```python
from build123d import *

# Parameters (mm, degrees)
CUT_EXTRUDE2_REACH = 19.55
CIRPATTERN1_COUNT  = 12


with BuildPart() as part:
    # Sketch1 → Revolve1 (revolve)
    with BuildSketch(Plane.XY, mode=Mode.PRIVATE) as revolve1_sk:
        Polygon((3.937, 47.625), (3.937, 55.894079216), (0.8255, 55.894079216), (0.8255, 51.371485268), (2.7305, 51.371485268), (2.7305, 47.625), align=None)
    revolve(revolve1_sk.sketch.rotate(Axis((6.7945, 45.4025, 0), (0, 1, 0)), 270), axis=Axis((6.7945, 45.4025, 0), (0, 1, 0)))

    # Sketch2 → Cut-Extrude2 (cut, up to next)
    with BuildSketch(Plane(origin=(-1.519613368, 55.894079216, 0), x_dir=(-1, 0, 0), z_dir=(0, 1, 0)), mode=Mode.PRIVATE) as cut_extrude2_sk1:
        with BuildLine():
            Line((-3.694980373, 0.479092135), (-2.424980373, 0.973177048))
            ThreePointArc((-2.424980373, 0.973177048), (-2.345113368, 0), (-2.424980373, -0.973177048))
            Line((-2.424980373, -0.973177048), (-3.694980373, -0.479092135))
            Line((-3.694980373, -0.479092135), (-3.694980373, 0.479092135))
        make_face()
    cut_extrude2_tool1 = extrude(cut_extrude2_sk1.sketch, amount=-CUT_EXTRUDE2_REACH, mode=Mode.PRIVATE) & part.part
    cut_extrude2 = cut_extrude2_tool1.solids().sort_by_distance((1.436663, 55.894079, 0))[0]
    add(cut_extrude2, mode=Mode.SUBTRACT)

    # CirPattern1: Cut-Extrude2 ×12 about axis
    cirpattern1_axis = Axis((6.7945, 0, 0), (0, 1, 0))
    for i in range(1, CIRPATTERN1_COUNT):
        add(cut_extrude2.rotate(cirpattern1_axis, i * 360 / CIRPATTERN1_COUNT), mode=Mode.SUBTRACT)


solid = part.part
```
The model under review builds one solid part; all positions refer to its coordinate system, in mm. A direction names the side the tool comes from. Round coordinates to 2 decimals unless told otherwise and drop trailing zeros. Loops run counter-clockwise (first coordinate to the right, second up) from the corner with the lowest first, then second, coordinate; pieces in that order, holes last. Notation, with made-up numbers: M 53,35 L 82,35 A22 cw 82,42 Z; hole C 42,-16.75 d9. An arc over 180 degrees is marked long. Write item = value, one per line.
Item 1: Take a section at C-C on z = 3.5. Write out the cut boundary in (x, y) (3 decimals).
Return value:
outline = M 2.412,51.371 L 4.729,51.371 L 4.729,47.625 L 8.86,47.625 L 8.86,51.371 L 11.177,51.371 L 11.177,55.894 L 2.412,55.894 Z
Item 2: Take a section at D-D on y = 49.75. Write out the cut boundary in (x, z) (1 decimal).
Return value:
outline = C 6.8,0 d8.1; hole C 6.8,0 d5.7
Item 3: Insertion check: P1, Ø1.5, axis at x = 4, y = 54, coming from the +Z side; P2, Ø2, axis at x = 4.5, y = 50.5, coming from the -Z side; P3, Ø1, axis at x = 2.5, z = -3, coming from the -Y side. Each pin has a flat end and moves straight along its axis. Give the tip position at first contact, or say it passes through.
Return value:
P1 = 5.61
P2 = -5.69
P3 = 51.37
Item 4: Take a section at A-A on z = 0. Write out the cut boundary in (x, y) (1 decimal), then the cut area to 3 significant figures.
Return value:
outline = M 2.2,51.4 L 2.7,51.4 L 2.7,47.6 L 3.9,47.6 L 3.9,55.9 L 2.2,55.9 Z; M 9.7,47.6 L 10.9,47.6 L 10.9,51.4 L 11.4,51.4 L 11.4,55.9 L 9.7,55.9 Z
area = 25.0 mm2
Item 5: For line 1 (X direction, y = 52, z = 4.5); line 2 (X direction, y = 51.5, z = 0); line 3 (X direction, y = 49.5, z = 0), list the stretches that pass through material, from the lowest coordinate up. Write a range as [from, to].
Return value:
line_1 = [2.87, 3.15], [4.86, 8.73], [10.44, 10.72]
line_2 = [2.18, 3.94], [9.65, 11.41]
line_3 = [2.73, 3.94], [9.65, 10.86]
Item 6: Take a section at B-B on x = 7.5. Write out the cut boundary in (y, z) (3 decimals).
Return value:
outline = M 47.625,-4.002 L 51.371,-4.002 L 51.371,-5.201 L 55.894,-5.201 L 55.894,-2.769 L 47.625,-2.769 Z; M 47.625,2.769 L 55.894,2.769 L 55.894,5.201 L 51.371,5.201 L 51.371,4.002 L 47.625,4.002 Z
Item 7: The part is to be moulded in two halves that separate along Z. For faces 1 (the flat face through (7, 54, 4.619)), 2 (the flat face through (3, 51.371, 2)), 3 (the flat face through (2.601, 53.664, -3.263)), say which applies: released by +Z, released by -Z, zero draft, split by the parting line, or undercut.
Return value:
face_1 = released by +Z
face_2 = zero draft
face_3 = undercut
Item 8: Machinability: for faces 4 (the flat face through (2.61, 53.66, 3.25)), 5 (the cylindrical face through (10.762, 49.472, 0.881)), 6 (the flat face through (11.414, 54, 0)), 7 (the flat face through (4.491, 53.664, -4.004)), 8 (the flat face through (10.058, 53.664, -4.193)), which of the approach directions +Z, -Z, +X, -X, +Y, -Y give a long, thin tool a straight path to every point of the face, cutting with its end or side? Answer none if there is none.
Return value:
face_4 = -X, +Y, -Y
face_5 = -Y
face_6 = +X, +Y, -Y
face_7 = +Y, -Y
face_8 = -Z, +Y, -Y
